Model file for the job. Use its own axes, mm. A direction names the side the tool comes from. Give positions to 0.01 mm unless a question says otherwise; leave off trailing zeros. Write each loop counter-clockwise with the first axis right and the second up, starting at its lowest first coordinate (ties: lowest second). Pieces come first, ordered by that corner, then holes. Notation, with made-up numbers: (9, -26) - (19, -26) arc R22 ccw to (19, 11) - close; hole circle Ø1 at (59.25, 13). An arc over 180 degrees is marked (long way). One line per item, written item: value. Start each with the question number.
(1) Drop flat-ended pins along their axis: P1, Ø12, axis at x = 1, y = 6.5, coming from the -Z side; P2, Ø8, axis at x = 4.5, y = 3, coming from the +Z side; P3, Ø2, axis at x = -3.5, y = 12, coming from the -Z side; P4, Ø1.5, axis at x = -12, z = 331.5, coming from the -Y side. Give the stop position or say it passes through.
(2) Cut at A-A, the plane z = 975.5. List the corners of the cut face in (x, y).
(3) 3-axis set-ups, long thin cutter, end or side, ignore diameter. For faces 1 (the face through (-12, 0, 515)), 2 (the face through (15, 0, 544)): which of +Z, -Z, +X, -X, +Y, -Y reach the whole face in a straight line?
(4) Mould opens along X. For faces 3 (the face through (0.07, -12.29, 1054.72)), 4 (the face through (12, 0, 541)), 5 (the face through (0, -12, 538)), 6 (the face through (0, -15, 538)) say: pulls with the +X half, pulls with the -X half, needs draft (parallel to the pull), parting line crosses it, or undercut.
(5) Probe L1, parallel to X at y = 7.5, z = 64; L2, parallel to X at y = 11.5, z = 860.5. List the from-to ranges inside material, lowest first.
(6) Cut at C-C, the plane x = -0.5. List the corners of the cut face in (y, z), and give its area (3 significant figures).
(7) Cut at B-B, the plane y = -2.5. List the corners of the cut face in (x, z), and give its area (3 significant figures).
Autodesk Inventor part; units mm, degrees
ref_plane "Start Plane" through (0, 0, 10.2298) normal (0, 0, 1) x (1, 0, 0)
ref_plane "End Plane" through (0, 0, 1092.7916) normal (0, 0, 1) x (1, 0, 0)
ref_plane "Work Plane4" through (10.6788, 0, 1081.7726) normal (-0.931, 0, 0.3651) x (0.3651, 0, 0.931)
ref_plane "Start Plane" through (0, 0, 10.2298) normal (0, 0, 1) x (1, 0, 0)
ref_plane "End Plane" through (0, 0, 1092.7916) normal (0, 0, 1) x (1, 0, 0)
sketch "Sketch" plane through (0, 0, 0) normal (0, 0, 1) x (1, 0, 0)
  line L0 (-15, -9) -> (-15, 9)
  line L1 (-9, 15) -> (9, 15)
  line L2 (15, 9) -> (15, -9)
  line L3 (9, -15) -> (-9, -15)
  arc A0 (-15, -9) -> (-9, -15) centre (-9, -9) ccw
  arc A1 (-9, 15) -> (-15, 9) centre (-9, 9) ccw
  arc A2 (15, 9) -> (9, 15) centre (9, 9) ccw
  arc A3 (9, -15) -> (15, -9) centre (9, -9) ccw
  arc A4 (-9, 12) -> (-12, 9) centre (-9, 9) ccw
  line L4 (-9, 12) -> (9, 12)
  arc A5 (12, 9) -> (9, 12) centre (9, 9) ccw
  line L5 (12, 9) -> (12, -9)
  arc A6 (9, -12) -> (12, -9) centre (9, -9) ccw
  line L6 (9, -12) -> (-9, -12)
  arc A7 (-12, -9) -> (-9, -12) centre (-9, -9) ccw
  line L7 (-12, -9) -> (-12, 9)
  line L8 (0, 22.7397) -> (0, -22.7397) construction
  line L9 (-22.7397, 0) -> (22.7397, 0) construction
  dimension "d7" = 6
  dimension "d10" = 30
  dimension "d11" = 30
  dimension "d12" = 3
  dimension "d15" = 15
  dimension "d16" = 15
extrude "Body" add sketch "Sketch" along normal up to surface (1082.5618 mm away) from surface at 10.2298
sketch "Sketch3" plane through (0, 0, 0) normal (0, 0, 1) x (1, 0, 0)
  line L0 (0, 0) -> (10, 0)
ref_plane "Work Plane3" through (0, 0, 0) normal (0, -1, 0) x (1, 0, 0)
ref_plane "Work Plane4" through (10.6788, 0, 1081.7726) normal (-0.931, 0, 0.3651) x (0.3651, 0, 0.931)
split "Split1" plane through (10.6788, 0, 1081.7726) removes the side toward (-0.931, 0, 0.3651)
ref_plane "Work Plane5" through (-358.4247, 9, 140.5587) normal (-0.931, 0, 0.3651) x (0.3651, 0, 0.931)
split "Split2" plane through (-358.4247, 9, 140.5587) removes the side toward (-0.931, 0, 0.3651)
ref_plane "Work Plane6" through (13.8551, 0, 10.6788) normal (-0.3651, 0, -0.931) x (-0.931, 0, 0.3651)
split "Split3" plane through (13.8551, 0, 10.6788) removes the side toward (-0.3651, 0, -0.931)
sketch "Sketch4" plane through (0, 0, 0) normal (0, -1, 0) x (1, 0, 0)
  line L0 (-2, 10.2298) -> (12, 10.2298)
  line L1 (-2, 1092.7916) -> (12, 1092.7916)
  dimension "d18" = 1082.5618
equation "\"d7\" = G_IR"
equation "\"d10\" = G_H"
equation "\"d11\" = G_W"
equation "\"d12\" = G_T"
equation "\"d15\" = 0.5 * d10"
equation "\"d16\" = 0.5 * d11"
equation "\"d3\" = G_L"
equation "\"G_W\" = 30"
equation "\"G_H\" = 30"
equation "\"G_T\" = 3"
equation "\"G_IR\" = 6"
equation "\"G_L\" = d18"
equation "\"G_OFFSET_START\" = -10.22982"
equation "\"G_OFFSET_END\" = -2.83604"
equation "\"d13\" = -G_OFFSET_START"
equation "\"d14\" = G_OFFSET_END + B_L"
equation "\"B_L\" = 1095.62767"
properties part number "DIN EN 10219-2 - 30 x 30 x 3  - 1082.56" material "Steel, Mild"
Answers follow:
1. P1: stops at z = 14.78
1. P2: passes through
1. P3: stops at z = 17.09
1. P4: stops at y = -14.56
2. outline: (-15, -9) arc R6 ccw to (-9, -15) - (9, -15) arc R6 ccw to (15, -9) - (15, 9) arc R6 ccw to (9, 15) - (-9, 15) arc R6 ccw to (-15, 9) - close; hole (-12, -9) arc R3 ccw to (-9, -12) - (9, -12) arc R3 ccw to (12, -9) - (12, 9) arc R3 ccw to (9, 12) - (-9, 12) arc R3 ccw to (-12, 9) - close
3. face 1: +Z, -Z
3. face 2: +Z, -Z, +X, +Y, -Y
4. face 3: pulls with the -X half
4. face 4: undercut
4. face 5: undercut
4. face 6: needs draft
5. L1: x = -15 to -12, 12 to 15
5. L2: x = -14.45 to -10.66, 10.66 to 14.45
6. outline: (-15, 16.31) - (-12, 16.31) - (-12, 1053.26) - (-15, 1053.26) - close; (12, 16.31) - (15, 16.31) - (15, 1053.26) - (12, 1053.26) - close
6. area: 6,220 mm²
7. outline: (-15, 21.99) - (-12, 20.82) - (-12, 1023.94) - (-15, 1016.29) - close; (12, 11.41) - (15, 10.23) - (15, 1092.79) - (12, 1085.14) - close
7. area: 6,230 mm²
